from build123d import *

# Parameters (mm, degrees)
F1_DEPTH = 127
F3_DEPTH = 38.1
F5_DEPTH = 273.05
F6_R     = 12.7
F7_DEPTH = 38.1


with BuildPart() as f1:
    # F0 (on Front) → F1 (new body)
    with BuildSketch(Plane.XZ):
        Polygon((0, 82.55), (0, 0), (304.8, 0), (304.8, 101.6), (266.7, 101.6), (266.7, 38.1), (31.75, 38.1), (31.75, 101.6), (19.05, 101.6), align=None)
    extrude(amount=F1_DEPTH)

    # F2 (on face) → F3 (cut)
    with BuildSketch(Plane.YZ.offset(304.8)):
        with BuildLine():
            Line((-127, 101.6), (-127, 50.8))
            Line((-127, 50.8), (-111.125, 50.8))
            Line((-111.125, 50.8), (-85.497045, 88.9))
            ThreePointArc((-85.497045, 88.9), (-76.2, 98.197045), (-63.5, 101.6))
            Line((-63.5, 101.6), (-127, 101.6))
        make_face()
        with BuildLine():
            Line((0, 101.6), (-63.5, 101.6))
            ThreePointArc((-63.5, 101.6), (-50.8, 98.197045), (-41.502955, 88.9))
            Line((-41.502955, 88.9), (-15.875, 50.8))
            Line((-15.875, 50.8), (0, 50.8))
            Line((0, 50.8), (0, 101.6))
        make_face()
    extrude(amount=-F3_DEPTH, mode=Mode.SUBTRACT)

    # F4 (on face) → F5 (cut)
    with BuildSketch(Plane.YZ.offset(304.8)):
        Polygon((-76.2, 16.51), (-76.2, 0), (-50.8, 0), (-50.8, 16.51), (-31.75, 16.51), (-31.75, 29.21), (-50.8, 29.21), (-50.8, 38.1), (-76.2, 38.1), (-76.2, 29.21), (-95.25, 29.21), (-95.25, 16.51), align=None)
    extrude(amount=-F5_DEPTH, mode=Mode.SUBTRACT)

    # F6 (on face) → F7 (cut)
    with BuildSketch(Plane.YZ.offset(304.8)):
        with Locations((-63.5, 82.55)):
            Circle(F6_R)
    extrude(amount=-F7_DEPTH, mode=Mode.SUBTRACT)


solid = f1.part
Work out the finished part from the listing and answer in its coordinate system (mm). A direction names the side the tool comes from. Give positions to 0.01 mm unless a question says otherwise; leave off trailing zeros. Order: outer loops, then holes, each group sorted by start corner. A loop starts at its lowest first (then second) coordinate and runs counter-clockwise, first axis right, second up. Notation, with made-up numbers: (-13, 63.5) - (-8, 63.5) arc R22 ccw to (-8, 90.5) - close; hole circle Ø8 at (41, 53.25). An arc over 180 degrees is marked (long way). Answer as CSV lines item,"result". Start each with the question number.
Q1. The part is cut by section C-C (z = 77.5). Write down the section's boundary in (x, y), then the cut area to 3 significant figures.
Q2. For faces 1 (the face through (151, -25, 38.1)), 2 (the face through (286, -8, 50.8)), 3 (the face through (170, -86, 16.51)), 4 (the face through (286, -119, 50.8)), determine the directions among +Z, -Z, +X, -X, +Y, -Y from which every point of the face is accessible in a straight line to the end or side of a thin tool.
Q3. The part is cut by section B-B (y = -117). Write down the section's boundary in (x, z), then the cut area to 3 significant figures.
Q4. The mould has two halves that part along Z. Classify faces 5 (the face through (286, -63, 38.1)), 6 (the face through (170, -41, 16.51)), 7 (the face through (0, -63, 42)): +Z half, -Z half, draft (parallel to the pull), parting line (faces both ways), or undercut.
Q5. Find the intervals of material crossed by L1, parallel to X at y = -37, z = 51; L2, parallel to Z at x = 289, y = -63.5; L3, parallel to Y at x = 41, z = 24.5, in increasing order. Write a range as [from, to].
Q6. The part is cut by section D-D (x = 270). Write down the section's boundary in (y, z) (3 decimals).
Q7. The part is cut by section A-A (x = 128.5). Write down the section's boundary in (y, z).
Q8. Given pin 1 Ø5 at (x, y) = (284, -7.5) entering from +Z; pin 2 Ø15 at (x, y) = (224.5, -83) entering from +Z; pin 3 Ø15 at (y, z) = (-63.5, 82.55) entering from +X, each flat-ended and moving along its own axis, determine where each tip first touches the part or whether it passes through.
Check result:
1,outline,"(0, -127) - (31.75, -127) - (31.75, 0) - (0, 0) - close; (266.7, -93.17) - (304.8, -93.17) - (304.8, -75.15) - (266.7, -75.15) - close; (266.7, -51.85) - (304.8, -51.85) - (304.8, -33.83) - (266.7, -33.83) - close"
1,area,"5,400 mm²"
2,face 1,"+Z, +Y, -Y"
2,face 2,"+Z, +X, +Y"
2,face 3,"+X"
2,face 4,"+Z, +X, -Y"
3,outline,"(0, 0) - (304.8, 0) - (304.8, 50.8) - (266.7, 50.8) - (266.7, 38.1) - (31.75, 38.1) - (31.75, 101.6) - (19.05, 101.6) - (0, 82.55) - close"
3,area,"13,900 mm²"
4,face 5,"-Z half"
4,face 6,"undercut"
4,face 7,"draft"
5,L1,"x = [0, 31.75], [266.7, 304.8]"
5,L2,"z = [38.1, 69.85], [95.25, 101.6]"
5,L3,"y = [-127, -95.25], [-31.75, 0]"
6,outline,"(-127, 0) - (-76.2, 0) - (-76.2, 16.51) - (-95.25, 16.51) - (-95.25, 29.21) - (-76.2, 29.21) - (-76.2, 38.1) - (-50.8, 38.1) - (-50.8, 29.21) - (-31.75, 29.21) - (-31.75, 16.51) - (-50.8, 16.51) - (-50.8, 0) - (0, 0) - (0, 50.8) - (-15.875, 50.8) - (-41.503, 88.9) arc R25.4 ccw to (-63.5, 101.6) arc R25.4 ccw to (-85.497, 88.9) - (-111.125, 50.8) - (-127, 50.8) - close; hole circle Ø25.4 at (-63.5, 82.55)"
7,outline,"(-127, 0) - (-76.2, 0) - (-76.2, 16.51) - (-95.25, 16.51) - (-95.25, 29.21) - (-76.2, 29.21) - (-76.2, 38.1) - (-127, 38.1) - close; (-50.8, 0) - (0, 0) - (0, 38.1) - (-50.8, 38.1) - (-50.8, 29.21) - (-31.75, 29.21) - (-31.75, 16.51) - (-50.8, 16.51) - close"
8,pin 1,"stops at z = 50.8"
8,pin 2,"stops at z = 38.1"
8,pin 3,"stops at x = 31.75"
